Autodesk Inventor part; units mm, degrees
ref_plane "YZ Plane" through (0, 0, 0) normal (1, 0, 0) x (0, 1, 0)
ref_plane "XZ Plane" through (0, 0, 0) normal (0, 1, 0) x (-1, 0, 0)
ref_plane "XY Plane" through (0, 0, 0) normal (0, 0, 1) x (1, 0, 0)
sketch "Sketch1" plane through (0, 0, 0) normal (0, 0, 1) x (1, 0, 0)
  circle A0 centre (0, 0) radius 47.371
  dimension "d0" = 94.742
extrude "Extrusion1" add sketch "Sketch1" along normal blind 40.64
sketch "Sketch2" plane through (0, 0, 0) normal (0, 0, -1) x (-1, 0, 0)
  circle A0 centre (0, 0) radius 42.8625
  dimension "d4" = 85.725
extrude "Extrusion2" cut sketch "Sketch2" against normal blind 31.75
sketch "Sketch6" plane through (0, 0, 40.64) normal (0, 0, 1) x (1, 0, 0)
  circle A0 centre (0, 0) radius 47.371
  circle A1 centre (0, 0) radius 19.05
  line L0 (0, 19.05) -> (0, 0) construction
  dimension "d24" = 38.1
hole "Hole3" at (0, 19.05, 40.64) direction (0, 0, -1) diameter 3.9624 depth 25.4 tip angle 118
pattern_circular "Circular Pattern1" count 5 over 360 about axis through (0, 0, 0) along (0, 0, 1) of "Hole3"
sketch "Sketch7" plane through (0, 0, 40.64) normal (0, 0, 1) x (1, 0, 0)
  circle A0 centre (0, 0) radius 47.371
  circle A1 centre (0, 0) radius 3.175
  dimension "d37" = 6.35
extrude "Extrusion4" add sketch "Sketch7" along normal blind 25.4 contours A1
properties part number "Aluminum mold support"
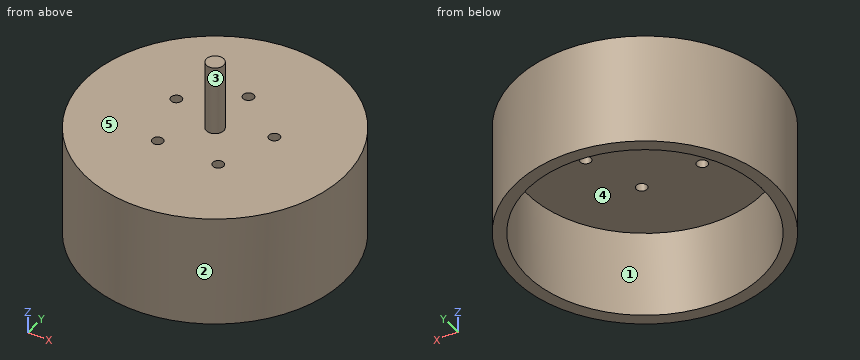
Work out the finished part from the listing and answer in its coordinate system (mm). Face numbers are marked on the shaded views. A direction names the side the tool comes from. Give positions to 0.01 mm unless a question says otherwise; leave off trailing zeros. Write each loop counter-clockwise with the first axis right and the second up, starting at its lowest first coordinate (ties: lowest second). Pieces come first, ordered by that corner, then holes. Notation, with made-up numbers: M 13,11.5 L 17,11.5 A27 cw 17,32.5 Z; hole C -18,-32 d1. An arc over 180 degrees is marked long. Answer as CSV lines item,"result".
Q1. Given P1, Ø5, axis at x = 18.12, y = 5.89, coming from the -Z side; P2, Ø2, axis at y = 26.5, z = 28, coming from the +X side; P3, Ø4, axis at x = 22, z = 18.5, coming from the -Y side, each flat-ended and moving along its own axis, determine where each tip first touches the part or whether it passes through.
A:
P1,"stops at z = 31.75"
P2,"stops at x = 39.92"
P3,"stops at y = -42.94"
Q2. A cutting plane is placed at C-C on z = 26. Write down the section's boundary in (x, y) (1 decimal), plus the area to 3 significant figures.
A:
outline,"C 0,0 d94.7; hole C 0,0 d85.7"
area,"1,280 mm²"
Q3. A tool of negligible diameter and unlimited length cuts with its end or side. For the marked faces 1 and 2, from which of +Z, -Z, +X, -X, +Y, -Y can it reach the whole face along a straight path? Write none if from no direction.
A:
face 1,"-Z"
face 2,"+Z, -Z"
Q4. Find the intervals of material crossed by probe 1 along Z at (x, y) = (14, -12); probe 2 along X at (y, z) = (11.5, 12.5); probe 3 along X at (y, z) = (7, 14), in increasing order. Write a range as [from, to].
A:
probe 1,"z = [31.75, 40.64]"
probe 2,"x = [-45.95, -41.29], [41.29, 45.95]"
probe 3,"x = [-46.85, -42.29], [42.29, 46.85]"
Q5. The mould has two halves that part along Y. Classify the marked faces 3, 4 and 5: +Y half, -Y half, draft (parallel to the pull), parting line (faces both ways), or undercut.
A:
face 3,"parting line"
face 4,"undercut"
face 5,"draft"
Q6. A cutting plane is placed at B-B on y = 19.05. Write down the section's boundary in (x, z).
A:
outline,"M -43.37,0 L -38.4,0 L -38.4,31.75 L -1.98,31.75 L -1.98,40.64 L -43.37,40.64 Z; M 1.98,31.75 L 38.4,31.75 L 38.4,0 L 43.37,0 L 43.37,40.64 L 1.98,40.64 Z"
